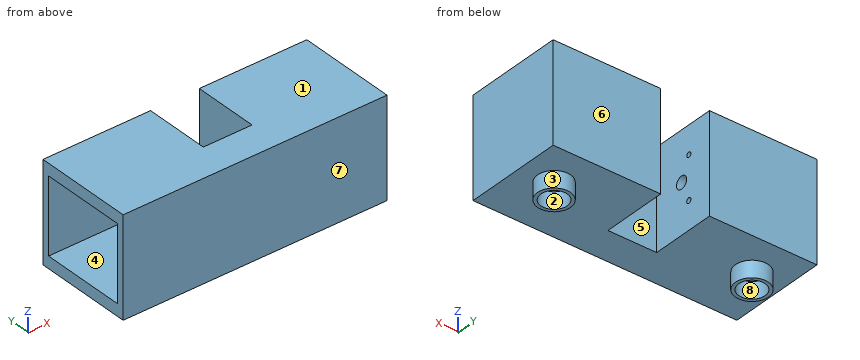
from build123d import *

# Parameters (mm, degrees)
SKICA1_W                 = 30
SKICA1_H                 = 30
P_IDAT_VYSUNUT_M1_DEPTH  = 40
SKICA2_W                 = 14.772421132
SKICA2_H                 = 61.833184582
ODEBRAT_VYSUNUT_M1_DEPTH = 180
SKICA3_W                 = 22.785077148
SKICA3_H                 = 25.847285536
ODEBRAT_VYSUNUT_M2_DEPTH = 30
SKICA4_R                 = 0.794930896
SKICA4_R_2               = 0.758797673
SKICA4_R_3               = 1.053455412
SKICA4_R_4               = 0.975597008
ODEBRAT_VYSUNUT_M3_DEPTH = 60
SKICA5_R                 = 1.886179275
ODEBRAT_VYSUNUT_M4_DEPTH = 30
SKICA6_R                 = 5
SKICA6_R_2               = 4
P_IDAT_VYSUNUT_M2_DEPTH  = 5


with BuildPart() as part:
    # Skica1 → Přidat vysunutím1 (new body, symmetric)
    with BuildSketch(Plane(origin=(0, 0, 0), x_dir=(0, 0, -1), z_dir=(1, 0, 0))):
        Rectangle(SKICA1_W, SKICA1_H)
    extrude(amount=P_IDAT_VYSUNUT_M1_DEPTH, both=True)

    # Skica2 → Odebrat vysunutím1 (cut)
    with BuildSketch(Plane(origin=(0, 0, -15), x_dir=(-1, 0, 0), z_dir=(0, 0, -1))):
        with Locations((0, 26.170702713)):
            Rectangle(SKICA2_W, SKICA2_H)
    extrude(amount=-ODEBRAT_VYSUNUT_M1_DEPTH, mode=Mode.SUBTRACT)

    # Skica3 → Odebrat vysunutím2 (cut)
    with BuildSketch(Plane.ZY.offset(40)):
        Rectangle(SKICA3_W, SKICA3_H)
    extrude(amount=-ODEBRAT_VYSUNUT_M2_DEPTH, mode=Mode.SUBTRACT)

    # Skica4 → Odebrat vysunutím3 (cut)
    with BuildSketch(Plane(origin=(-7.386210566, 0, 0), x_dir=(0, 0, -1), z_dir=(1, 0, 0))):
        with Locations((6.506049624, 7.292174822)):
            Circle(SKICA4_R)
        with Locations((-6.501910486, 7.292174822)):
            Circle(SKICA4_R_2)
        with Locations((-6.285111151, -9.654306544)):
            Circle(SKICA4_R_3)
        with Locations((6.506049624, -9.87110588)):
            Circle(SKICA4_R_4)
    extrude(amount=-ODEBRAT_VYSUNUT_M3_DEPTH, mode=Mode.SUBTRACT)

    # Skica5 → Odebrat vysunutím4 (cut)
    with BuildSketch(Plane.ZY.offset(10)):
        with Locations((0, 4.56487451)):
            Circle(SKICA5_R)
    extrude(amount=-ODEBRAT_VYSUNUT_M4_DEPTH, mode=Mode.SUBTRACT)

    # Skica6 → Přidat vysunutím2 (add)
    with BuildSketch(Plane(origin=(0, 0, -15), x_dir=(-1, 0, 0), z_dir=(0, 0, -1))):
        with Locations((-30, 3)):
            Circle(SKICA6_R)
        with Locations((-30, 3)):
            Circle(SKICA6_R_2, mode=Mode.SUBTRACT)
    p_idat_vysunut_m2 = extrude(amount=P_IDAT_VYSUNUT_M2_DEPTH)

    # Zrcadlit1: Přidat vysunutím2 across plane
    add(p_idat_vysunut_m2.mirror(Plane(origin=(0, 0, 0), x_dir=(0, 0, 1), z_dir=(1, 0, 0))))


solid = part.part
Can you work these out from the model? Positions are in its coordinate system, mm. Face numbers are marked on the shaded views. A direction names the side the tool comes from. Coordinates: 2 decimals unless noted, no trailing zeros. Order: outer loops, then holes, each group sorted by start corner. A loop starts at its lowest first (then second) coordinate and runs counter-clockwise, first axis right, second up. Notation, with made-up numbers: (-18.75, 36) - (30.25, 36) arc R32 ccw to (30.25, 73) - close; hole circle Ø6 at (79.25, 29). An arc over 180 degrees is marked (long way). Answer as a JSON object with one key per item and string values. Group by question number.
Q1. I need wall thicknesses on line 1 (Z direction, x = -12, y = -10); line 2 (X direction, y = 2.75, z = -7); line 3 (Y direction, x = 30, z = -16.55). Which ranges of each line are inside material? Lowest first, please. Write a range as from..to.
Q2. Imagine slicing it at C-C (z = 0). Please give me the cut outline in (x, y), and give its area (3 significant figures).
Q3. Will these pins go through, and if not, where does the flat tip stop? P1, Ø9, axis at x = -4, y = 2, coming from the -Z side; P2, Ø11.5, axis at y = -1.5, z = 0.5, coming from the -X side; P3, Ø1.1, axis at y = -9.5, z = 6, coming from the -X side; P4, Ø12, axis at y = -9, z = 1.5, coming from the -X side.
Q4. Imagine slicing it at B-B (x = -30). Please give me the cut outline in (y, z).
Q5. We'd pull the mould along Y, two halves only. Please class the marked faces 1, 2 and 3: +Y half, -Y half, draft (parallel to the pull), parting line (faces both ways), or undercut.
Q6. Imagine slicing it at D-D (z = 3.5). Please give me the cut outline in (x, y), and give its area (3 significant figures).
Q7. Imagine slicing it at A-A (y = 9.25). Please give me the cut outline in (x, z), and give its area (3 significant figures).
Q8. On a 3-axis mill with a long thin cutter (end or side, diameter ignored), from which of +Z, -Z, +X, -X, +Y, -Y can I reach the whole of each face in a straight line? I mean the marked faces 4, 5, 6, 7 and 8. Say none if no direction works.
Determined:
{
 "1": {"line 1": "z = -15..-11.39, 11.39..15", "line 2": "x = -10..-7.39, 7.39..40", "line 3": "y = -2..-1, 7..8"},
 "2": {"outline": "(-40, -15) - (40, -15) - (40, 15) - (7.39, 15) - (7.39, 6.45) - (20, 6.45) - (20, 2.68) - (7.39, 2.68) - (7.39, -4.75) - (-7.39, -4.75) - (-7.39, 2.68) - (-10, 2.68) - (-10, -12.92) - (-40, -12.92) - close; (-40, 12.92) - (-10, 12.92) - (-10, 6.45) - (-7.39, 6.45) - (-7.39, 15) - (-40, 15) - close", "area": "1,280 mm2"},
 "3": {"P1": "stops at z = -15", "P2": "stops at x = -10", "P3": "stops at x = -7.39", "P4": "stops at x = -40"},
 "4": {"outline": "(-15, -15) - (-2, -15) - (-2, -20) - (-1, -20) - (-1, -15) - (7, -15) - (7, -20) - (8, -20) - (8, -15) - (15, -15) - (15, 15) - (-15, 15) - close; hole (-12.92, -11.39) - (12.92, -11.39) - (12.92, 11.39) - (-12.92, 11.39) - close"},
 "5": {"face 1": "draft", "face 2": "undercut", "face 3": "parting line"},
 "6": {"outline": "(-40, -15) - (40, -15) - (40, 15) - (7.39, 15) - (7.39, -4.75) - (-7.39, -4.75) - (-7.39, 15) - (-40, 15) - (-40, 12.92) - (-10, 12.92) - (-10, -12.92) - (-40, -12.92) - close", "area": "1,330 mm2"},
 "7": {"outline": "(-40, -15) - (-7.39, -15) - (-7.39, 15) - (-40, 15) - (-40, 11.39) - (-10, 11.39) - (-10, -11.39) - (-40, -11.39) - close; (7.39, -15) - (40, -15) - (40, 15) - (7.39, 15) - close", "area": "1,270 mm2"},
 "8": {"face 4": "-X", "face 5": "+Z, -Z, +Y", "face 6": "+Z, -Z, +X, -X, +Y", "face 7": "+Z, -Z, +X, -X, -Y", "face 8": "-Z"}
}
